```python
from build123d import *

# Parameters (mm, degrees)
F1_DEPTH = 76.2
F2_W     = 31.1273433149
F2_H     = 14.4479367882
F3_DEPTH = 25.4
F4_W     = 25.4
F4_H     = 12.7
F5_DEPTH = 25.4


with BuildPart() as f1:
    # F0 (on Top) → F1 (new body)
    with BuildSketch(Plane.XY):
        Polygon((-39.3005906213, 21.688469161), (-39.3005906213, -41.811530839), (-26.6005906213, -41.811530839), (-26.6005906213, 8.988469161), (24.1994093787, 8.988469161), (24.1994093787, 21.688469161), align=None)
    extrude(amount=F1_DEPTH)

    # F2 (on face) → F3 (cut)
    with BuildSketch(Plane.YZ.offset(-26.6005906213)):
        with Locations((-26.2478591815, 7.2239683941)):
            Rectangle(F2_W, F2_H)
    extrude(amount=-F3_DEPTH, mode=Mode.SUBTRACT)

    # F4 (on face) → F5 (cut)
    with BuildSketch(Plane.YZ.offset(-26.6005906213)):
        with Locations((-29.111530839, 45.8086510956)):
            Rectangle(F4_W, F4_H)
    extrude(amount=-F5_DEPTH, mode=Mode.SUBTRACT)


solid = f1.part
```
Model file for the job. Use its own axes, mm. A direction names the side the tool comes from. Coordinates: 2 decimals unless noted, no trailing zeros. Loops run counter-clockwise (first coordinate to the right, second up) from the corner with the lowest first, then second, coordinate; pieces in that order, holes last. Notation, with made-up numbers: (-12.75, 81.5) -> (35.25, 81.5) arc R13 ccw to (35.25, 90.5) -> close; hole circle Ø4 at (39, 38). An arc over 180 degrees is marked (long way). Answer as a JSON object with one key per item and string values.
Q1. Cut at B-B (z = 44). List the corners of the cut face in (x, y), and give its area (3 significant figures).
Report:
{"outline": "(-39.3, -16.41) -> (-26.6, -16.41) -> (-26.6, 8.99) -> (24.2, 8.99) -> (24.2, 21.69) -> (-39.3, 21.69) -> close", "area": "1,130 mm2"}
Q2. 3-axis set-ups, long thin cutter, end or side, ignore diameter. For faces 1 (the flat face through (-26.601, -11, 46)), 2 (the flat face through (-33, -29, 52.159)), 3 (the flat face through (-33, -10.684, 7)): which of +Z, -Z, +X, -X, +Y, -Y reach the whole face in a straight line?
Report:
{"face 1": "+Z, -Z, +X, -Y", "face 2": "+X, -X, -Y", "face 3": "-Z, +X, -X, -Y"}
Q3. Flat gauge pins, fed straight in: P1, Ø15, axis at x = -2.5, z = 43, coming from the -Y side; P2, Ø6.5, axis at x = -33, z = 4.5, coming from the -Y side; P3, Ø4, axis at x = -33.5, y = -20.5, coming from the -Z side. Where does each tip first touch, or does it go through?
Report:
{"P1": "stops at y = 8.99", "P2": "stops at y = -10.68", "P3": "stops at z = 14.45"}
Q4. Pull direction Z, two halves, no side cores. Call faces 4 (the flat face through (-33, -26, 14.448)), 5 (the flat face through (-33, -16.412, 46)), 6 (the flat face through (-22, 12, 76.2)), 7 (the flat face through (-2, 8.988, 38)): released by +Z, released by -Z, zero draft, split by the parting line, or undercut.
Report:
{"face 4": "released by -Z", "face 5": "undercut", "face 6": "released by +Z", "face 7": "zero draft"}
Q5. Probe probe 1 along Z at (x, y) = (-31.5, -19); probe 2 along Y at (x, z) = (10, 69); probe 3 along X at (y, z) = (8, 5). List the from-to ranges inside material, lowest first.
Report:
{"probe 1": "z = 14.45 to 39.46, 52.16 to 76.2", "probe 2": "y = 8.99 to 21.69", "probe 3": "x = -39.3 to -26.6"}
Q6. Cut at A-A (y = -34). List the corners of the cut face in (x, z), and give its area (3 significant figures).
Report:
{"outline": "(-39.3, 14.45) -> (-26.6, 14.45) -> (-26.6, 39.46) -> (-39.3, 39.46) -> close; (-39.3, 52.16) -> (-26.6, 52.16) -> (-26.6, 76.2) -> (-39.3, 76.2) -> close", "area": "623 mm2"}
Q7. Cut at C-C (x = -13.5). List the corners of the cut face in (y, z).
Report:
{"outline": "(8.99, 0) -> (21.69, 0) -> (21.69, 76.2) -> (8.99, 76.2) -> close"}
Q8. Cut at D-D (y = -3). List the corners of the cut face in (x, z), and give its area (3 significant figures).
Report:
{"outline": "(-39.3, 0) -> (-26.6, 0) -> (-26.6, 76.2) -> (-39.3, 76.2) -> close", "area": "968 mm2"}
